```python
from build123d import *

# Parameters (mm, degrees)
SKETCH1_R               = 12.5
BOSS_EXTRUDE1_DEPTH     = 11
CUT_EXTRUDE1_DEPTH      = 21.820662814
CUT_EXTRUDE1_DEPTH_BACK = 21.820662814
SKETCH2_R               = 2
SKETCH3_R               = 11.5
SKETCH3_R_2             = 5
CUT_EXTRUDE2_DEPTH      = 0.5


with BuildPart() as part:
    # Sketch1 → Boss-Extrude1 (new body)
    with BuildSketch(Plane(origin=(0, 0, 0), x_dir=(1, 0, 0), z_dir=(0, 1, 0))):
        with Locations(Location((0, 0, 0), (0, 0, 270))):
            Circle(SKETCH1_R)
    extrude(amount=BOSS_EXTRUDE1_DEPTH)

    # Sketch2 → Cut-Extrude1 (cut, two sides: drawn at the far end of the back side and taken through both)
    with BuildSketch(Plane(origin=(0, 11, 0), x_dir=(1, 0, 0), z_dir=(0, 1, 0)).offset(-CUT_EXTRUDE1_DEPTH_BACK)):
        with Locations(Location((0, 0, 0), (0, 0, 270))):
            Circle(SKETCH2_R)
    extrude(amount=CUT_EXTRUDE1_DEPTH + CUT_EXTRUDE1_DEPTH_BACK, mode=Mode.SUBTRACT)

    # Sketch3 → Cut-Extrude2 (cut)
    with BuildSketch(Plane.XZ):
        with Locations(Location((0, 0, 0), (0, 0, 270))):
            Circle(SKETCH3_R)
        with Locations(Location((0, 0, 0), (0, 0, 270))):
            Circle(SKETCH3_R_2, mode=Mode.SUBTRACT)
    extrude(amount=-CUT_EXTRUDE2_DEPTH, mode=Mode.SUBTRACT)


solid = part.part
```
Model file for the job. Use its own axes, mm. A direction names the side the tool comes from. Give positions to 0.01 mm unless a question says otherwise; leave off trailing zeros. Write each loop counter-clockwise with the first axis right and the second up, starting at its lowest first coordinate (ties: lowest second). Pieces come first, ordered by that corner, then holes. Notation, with made-up numbers: (49.25, 16.5) -> (69.25, 16.5) arc R13 cw to (69.25, 35.5) -> close; hole circle Ø4 at (11.25, 80.25). An arc over 180 degrees is marked (long way). Use CSV: the item, a comma, the result in double quotes. Start each with the question number.
1) Cut at A-A on x = 0. List the corners of the cut face in (y, z).
2) Pin check, flat tips, straight feed: P1, Ø6, axis at y = 5, z = -8, coming from the -X side; P2, Ø2.5, axis at x = 0, z = 0, coming from the -Y side; P3, Ø2, axis at x = 6, y = 3, coming from the -Z side. Stop position of each tip, or through.
3) Cut at B-B on z = 0. List the corners of the cut face in (x, y).
4) Cut at D-D on x = 4.25. List the corners of the cut face in (y, z), plus the area to 3 significant figures.
5) Cut at C-C on y = 8.75. List the corners of the cut face in (x, z).
6) Tool access for faces 1 (the flat face through (-2, 0.5, -5)), 2 (the cylindrical face through (-2, 5, 0)): list every direction of +Z, -Z, +X, -X, +Y, -Y with a clear straight run to the whole face (end or side of a thin tool).
7) Drill centre lines: L1, parallel to X at y = 0.1, z = 0; L2, parallel to X at y = 5.5, z = 0; L3, parallel to Y at x = 5.75, z = 1. Where is each one in solid material? Low to high.
8) Two-plate mould, pull along Z, no slides. Class faces 3 (the cylindrical face through (-4.88, 0.25, 1.08)), 4 (the flat face through (-2.2, 0, -0.1)), 5 (the cylindrical face through (3.755, 5.423, 11.923)): released by +Z, released by -Z, zero draft, split by the parting line, or undercut.
Final values:
1,outline,"(0, -12.5) -> (11, -12.5) -> (11, -2) -> (0, -2) -> (0, -5) -> (0.5, -5) -> (0.5, -11.5) -> (0, -11.5) -> close; (0, 2) -> (11, 2) -> (11, 12.5) -> (0, 12.5) -> (0, 11.5) -> (0.5, 11.5) -> (0.5, 5) -> (0, 5) -> close"
2,P1,"stops at x = -11.46"
2,P2,"passes through"
2,P3,"stops at z = -11.46"
3,outline,"(-12.5, 0) -> (-11.5, 0) -> (-11.5, 0.5) -> (-5, 0.5) -> (-5, 0) -> (-2, 0) -> (-2, 11) -> (-12.5, 11) -> close; (2, 0) -> (5, 0) -> (5, 0.5) -> (11.5, 0.5) -> (11.5, 0) -> (12.5, 0) -> (12.5, 11) -> (2, 11) -> close"
4,outline,"(0, -11.76) -> (11, -11.76) -> (11, 11.76) -> (0, 11.76) -> (0, 10.69) -> (0.5, 10.69) -> (0.5, 2.63) -> (0, 2.63) -> (0, -2.63) -> (0.5, -2.63) -> (0.5, -10.69) -> (0, -10.69) -> close"
4,area,"251 mm2"
5,outline,"circle Ø25 at (0, 0); hole circle Ø4 at (0, 0)"
6,face 1,"-Y"
6,face 2,"+Y, -Y"
7,L1,"x = -12.5 to -11.5, -5 to -2, 2 to 5, 11.5 to 12.5"
7,L2,"x = -12.5 to -2, 2 to 12.5"
7,L3,"y = 0.5 to 11"
8,face 3,"undercut"
8,face 4,"zero draft"
8,face 5,"split by the parting line"
